Build history of the part. All positions in model axes, mm. A direction names the side the tool comes from. Coordinates: 2 decimals unless noted, no trailing zeros. Write each loop counter-clockwise with the first axis right and the second up, starting at its lowest first coordinate (ties: lowest second). Pieces come first, ordered by that corner, then holes.
```python
from build123d import *

# Parameters (mm, degrees)
EXTRUDE_2_DEPTH      = 10
FILLET_2_R           = 20
SKETCH_4_R           = 2.6
CUT_EXTRUDE_2_DEPTH  = 168.928556237
SKETCH_5_R           = 8.5
CUT_EXTRUDE_3_DEPTH  = 168.928556237
SKETCH_17_R          = 1.7
CUT_EXTRUDE_11_DEPTH = 10
SKETCH_18_R          = 2.1
CUT_EXTRUDE_12_DEPTH = 10


with BuildPart() as part:
    # 草图2 → 凸台-拉伸2 (new body)
    with BuildSketch(Plane(origin=(0, 0, 0), x_dir=(1, 0, 0), z_dir=(0, 1, 0))):
        Polygon((0, 50), (0, -50), (-90, -50), (-90, -30), (-160, -30), (-160, 30), (-90, 30), (-90, 50), align=None)
    extrude(amount=EXTRUDE_2_DEPTH)

    # 圆角2
    fillet_2_edges = [part.edges().sort_by_distance(p)[0] for p in [
        (-160, 5, 30),
        (-160, 5, -30),
    ]]
    fillet(fillet_2_edges, radius=FILLET_2_R)

    # 草图4 → 切除-拉伸2 (cut, through all)
    with BuildSketch(Plane(origin=(0, 10, 0), x_dir=(1, 0, 0), z_dir=(0, 1, 0))):
        with Locations(Location((-60, -40, 0), (0, 0, 270))):
            Circle(SKETCH_4_R)
        with Locations(Location((-80, -40, 0), (0, 0, 270))):
            Circle(SKETCH_4_R)
        with Locations(Location((-80, 40, 0), (0, 0, 270))):
            Circle(SKETCH_4_R)
        with Locations(Location((-60, 40, 0), (0, 0, 270))):
            Circle(SKETCH_4_R)
    extrude(amount=-CUT_EXTRUDE_2_DEPTH, mode=Mode.SUBTRACT)

    # 草图5 → 切除-拉伸3 (cut, through all)
    with BuildSketch(Plane.XZ):
        with Locations(Location((-45, 0, 0), (0, 0, 270))):
            Circle(SKETCH_5_R)
    extrude(amount=-CUT_EXTRUDE_3_DEPTH, mode=Mode.SUBTRACT)

    # 草图17 → 切除-拉伸11 (cut)
    with BuildSketch(Plane.XZ):
        with Locations(Location((-45, 16, 0), (0, 0, 270))):
            Circle(SKETCH_17_R)
        with Locations(Location((-45, -16, 0), (0, 0, 270))):
            Circle(SKETCH_17_R)
        with Locations(Location((-29, 0, 0), (0, 0, 270))):
            Circle(SKETCH_17_R)
        with Locations(Location((-61, 0, 0), (0, 0, 90))):
            Circle(SKETCH_17_R)
    extrude(amount=-CUT_EXTRUDE_11_DEPTH, mode=Mode.SUBTRACT)

    # 草图18 → 切除-拉伸12 (cut)
    with BuildSketch(Plane.XZ):
        with Locations(Location((-120, 12.5, 0), (0, 0, 270))):
            Circle(SKETCH_18_R)
        with Locations(Location((-132.5, 0, 0), (0, 0, 270))):
            Circle(SKETCH_18_R)
        with Locations(Location((-120, -12.5, 0), (0, 0, 270))):
            Circle(SKETCH_18_R)
        with Locations(Location((-107.5, 0, 0), (0, 0, 270))):
            Circle(SKETCH_18_R)
    extrude(amount=-CUT_EXTRUDE_12_DEPTH, mode=Mode.SUBTRACT)


solid = part.part
```
1. Saw through at A-A on x = -107.5. List the corners of the cut face in (y, z), plus the area to 3 significant figures.
Computed values:
outline: (0, -30) - (10, -30) - (10, -2.1) - (0, -2.1) - close; (0, 2.1) - (10, 2.1) - (10, 30) - (0, 30) - close
area: 558 mm2
2. Probe line 1 along X through (y, z) = (5.25, 0); line 2 along X through (y, z) = (5.5, 40); line 3 along Z through (x, y) = (-132.5, 4.75). List the from-to ranges inside material, lowest first.
Computed values:
line 1: x = -160 to -134.6, -130.4 to -109.6, -105.4 to -62.7, -59.3 to -53.5, -36.5 to -30.7, -27.3 to 0
line 2: x = -90 to -82.6, -77.4 to -62.6, -57.4 to 0
line 3: z = -30 to -2.1, 2.1 to 30
3. Saw through at D-D on z = -6. List the corners of the cut face in (x, y).
Computed values:
outline: (-160, 0) - (-51.02, 0) - (-51.02, 10) - (-160, 10) - close; (-38.98, 0) - (0, 0) - (0, 10) - (-38.98, 10) - close
4. Flat gauge pins, fed straight in: pin 1 (1.5 mm diameter, centred on x = -113, y = 5, fed in from -Z); pin 2 (5 mm diameter, centred on y = 3.5, z = -44.5, fed in from -X); pin 3 (3 mm diameter, centred on x = -121, y = 7, fed in from +Z). Where does each tip first touch, or does it go through?
Computed values:
pin 1: stops at z = -30
pin 2: stops at x = -90
pin 3: stops at z = 30
5. 3-axis set-ups, long thin cutter, end or side, ignore diameter. For faces 5 (the face through (-79, 0, -1)), 6 (the face through (-90, 5, -40)), 7 (the face through (-115, 5, 30)): which of +Z, -Z, +X, -X, +Y, -Y reach the whole face in a straight line?
Computed values:
face 5: +Z, -Z, +X, -X, -Y
face 6: -Z, -X, +Y, -Y
face 7: +Z, -X, +Y, -Y
6. Saw through at C-C on z = -40. List the corners of the cut face in (x, y).
Computed values:
outline: (-90, 0) - (-82.6, 0) - (-82.6, 10) - (-90, 10) - close; (-77.4, 0) - (-62.6, 0) - (-62.6, 10) - (-77.4, 10) - close; (-57.4, 0) - (0, 0) - (0, 10) - (-57.4, 10) - close
7. Saw through at B-B on y = 4. State how many separate pieces and enclosed holes the cut face has, plus the area to 3 significant figures.
Computed values:
separate pieces: 1
enclosed holes: 13
area: 12,600 mm2
8. Mould opens along X. For faces 1 (the face through (-46, 5, -50)), 2 (the face through (-122.05, 4.93, -12.04)), 3 (the face through (-46.5, 4.9, 15.2)), 4 (the face through (-90, 5, 40)) say: +X half, -X half, draft (parallel to the pull), parting line (faces both ways), or undercut.
Computed values:
face 1: draft
face 2: undercut
face 3: undercut
face 4: -X half
